Can you work these out from the model? Positions are in its coordinate system, mm. Coordinates: 2 decimals unless noted, no trailing zeros. Loops run counter-clockwise (first coordinate to the right, second up) from the corner with the lowest first, then second, coordinate; pieces in that order, holes last.
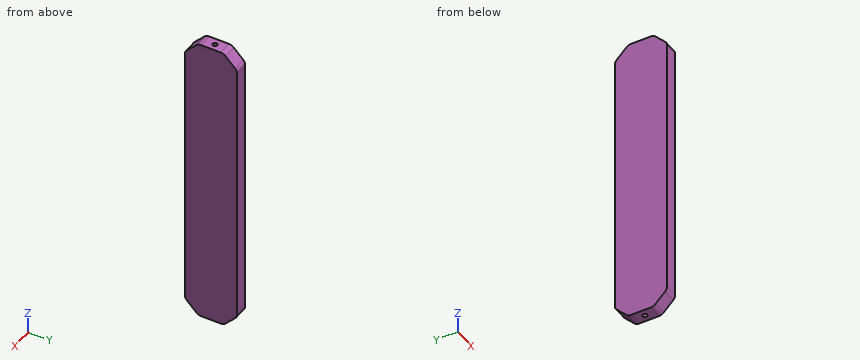
```python
from build123d import *

# Parameters (mm, degrees)
SKETCH1_W                        = 10
SKETCH1_H                        = 218
BOSS_EXTRUDE1_DEPTH              = 38
CUT_EXTRUDE1_DEPTH               = 11
FILLET1_R                        = 4.92
F_30_0_1285_DIAMETER_HOLE1_D     = 3.2639
F_30_0_1285_DIAMETER_HOLE1_DEPTH = 9.99998
F_30_0_1285_DIAMETER_HOLE1_TIP   = 0.980574487
F_30_0_1285_DIAMETER_HOLE2_D     = 3.2639
F_30_0_1285_DIAMETER_HOLE2_DEPTH = 9.906
F_30_0_1285_DIAMETER_HOLE2_TIP   = 0.980574487


with BuildPart() as part:
    # Sketch1 → Boss-Extrude1 (new body)
    with BuildSketch(Plane(origin=(0, 0, 0), x_dir=(1, 0, 0), z_dir=(0, 1, 0))):
        with Locations((5, 109)):
            Rectangle(SKETCH1_W, SKETCH1_H)
    extrude(amount=BOSS_EXTRUDE1_DEPTH)

    # Sketch3 → Cut-Extrude1 (cut, through all)
    with BuildSketch(Plane(origin=(0, 0, 0), x_dir=(0, 0, -1), z_dir=(1, 0, 0))):
        Polygon((218, 38), (208, 38), (218, 28.202041029), align=None)
        Polygon((218, 9.797958971), (218, 0), (208, 0), align=None)
        Polygon((0, 0), (10, 0), (0, 9.797958971), align=None)
        Polygon((0, 28.202041029), (0, 38), (10, 38), align=None)
    extrude(amount=CUT_EXTRUDE1_DEPTH, mode=Mode.SUBTRACT)

    # Fillet1
    fillet1_edges = [part.edges().sort_by_distance(p)[0] for p in [
        (5, 28.202041029, 0),
        (5, 38, -10),
        (5, 9.797958971, 0),
        (5, 0, -10),
        (5, 9.797958971, -218),
        (5, 0, -208),
        (5, 28.202041029, -218),
        (5, 38, -208),
    ]]
    fillet(fillet1_edges, radius=FILLET1_R)

    # #30 (0.1285) Diameter Hole1
    with Locations(Plane.XY):
        with Locations((5, 19)):
            Hole(F_30_0_1285_DIAMETER_HOLE1_D / 2, depth=F_30_0_1285_DIAMETER_HOLE1_DEPTH)
            with Locations((0, 0, -(F_30_0_1285_DIAMETER_HOLE1_DEPTH + F_30_0_1285_DIAMETER_HOLE1_TIP / 2))):  # 118° drill point
                Cone(0, F_30_0_1285_DIAMETER_HOLE1_D / 2, F_30_0_1285_DIAMETER_HOLE1_TIP, mode=Mode.SUBTRACT)

    # #30 (0.1285) Diameter Hole2
    with Locations(Plane(origin=(0, 0, -218), x_dir=(-1, 0, 0), z_dir=(0, 0, -1))):
        with Locations((-5, 19)):
            Hole(F_30_0_1285_DIAMETER_HOLE2_D / 2, depth=F_30_0_1285_DIAMETER_HOLE2_DEPTH)
            with Locations((0, 0, -(F_30_0_1285_DIAMETER_HOLE2_DEPTH + F_30_0_1285_DIAMETER_HOLE2_TIP / 2))):  # 118° drill point
                Cone(0, F_30_0_1285_DIAMETER_HOLE2_D / 2, F_30_0_1285_DIAMETER_HOLE2_TIP, mode=Mode.SUBTRACT)


solid = part.part
```
(1) If I drill on probe 1 along X at (y, z) = (19, -212); probe 2 along Y at (x, z) = (5, -210.25); probe 3 along Y at (x, z) = (5, -214.75), over which ranges is the centre line in solid material (lowest first)?
Check values:
probe 1: x = 0 to 3.37, 6.63 to 10
probe 2: y = 2.2 to 17.37, 20.63 to 35.8
probe 3: y = 6.61 to 17.37, 20.63 to 31.39
(2) I'm going to push a flat-ended pin straight in: pin 1 (2.5 mm diameter, centred on x = 5, y = 19, fed in from -Z). Where does the tip first touch, or does it pass through?
Check values:
pin 1: stops at z = -207.86
(3) I want a section at B-B on y = 4.5. Write out the boundary of the cut face in (x, z).
Check values:
outline: (0, -212.59) - (10, -212.59) - (10, -5.41) - (0, -5.41) - close
(4) I want a section at A-A on y = 32. Write out the boundary of the cut face in (x, z).
Check values:
outline: (0, -214.12) - (10, -214.12) - (10, -3.88) - (0, -3.88) - close
